from build123d import *

# Parameters (mm, degrees)
F2_T = -1
F3_R = 1


with BuildPart() as f1:
    # F0 (on Front) → F1 (revolve)
    with BuildSketch(Plane.XZ):
        Polygon((0, 9), (0, 0), (6.5, 0), (3.5, 9), align=None)
    revolve(axis=Axis((0, 0, 4.5), (0, 0, -1)))

    # F2
    f2_openings = [f1.faces().sort_by_distance(p)[0] for p in [
        (0, 0, 0),
    ]]
    offset(amount=F2_T, openings=f2_openings)

    # F3
    f3_edges = [f1.edges().sort_by_distance(p)[0] for p in [
        (-3.5, 0, 9),
    ]]
    fillet(f3_edges, radius=F3_R)


solid = f1.part
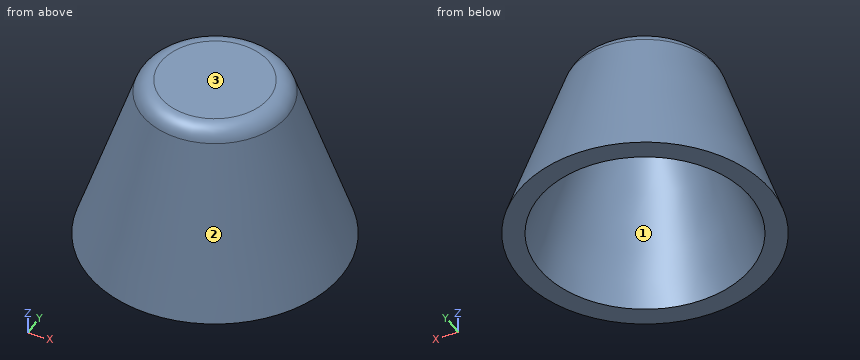
Could you check a few things on this model? Use its own coordinates, in mm. Face numbers are marked on the shaded views. Round coordinates to 2 decimals unless told otherwise and drop trailing zeros. Write each loop counter-clockwise with the first axis right and the second up, starting at its lowest first coordinate (ties: lowest second). Pieces come first, ordered by that corner, then holes. Notation, with made-up numbers: (39, -34.5) - (52, -34.5) arc R16 cw to (52, -8.5) - close; hole circle Ø7 at (-25.75, -1.5). An arc over 180 degrees is marked (long way). Use a Markdown table: item, result.
Q1. I want a section at A-A (x = 0). List the corners of the cut face in (y, z) for me.
Output values:
| item | result |
|---|---|
| outline | (-6.5, 0) - (-5.45, 0) - (-2.78, 8) - (2.78, 8) - (5.45, 0) - (6.5, 0) - (3.73, 8.32) arc R1 ccw to (2.78, 9) - (-2.78, 9) arc R1 ccw to (-3.73, 8.32) - close |
Q2. For pin 1 (1.5 mm diameter, centred on y = 1, z = 3.5, fed in from +X); pin 2 (1 mm diameter, centred on x = 5, z = 3, fed in from +Y); pin 3 (6 mm diameter, centred on x = -3.5, y = -2.5, fed in from +Z); pin 4 (1.7 mm diameter, centred on x = 1, y = 1.5, fed in from -Z), each with a flat end and sliding along its axis, tell me the tip position at first contact or that it passes through.
Output values:
| item | result |
|---|---|
| pin 1 | x = 5.52 |
| pin 2 | y = 3.22 |
| pin 3 | z = 9 |
| pin 4 | z = 8 |
Q3. Thinking about a two-plate mould opening in Y: for the marked faces 1, 2 and 3, which applies, released by +Y, released by -Y, zero draft, split by the parting line, or undercut?
Output values:
| item | result |
|---|---|
| face 1 | undercut |
| face 2 | split by the parting line |
| face 3 | zero draft |
Q4. I want a section at C-C (z = 1.25). List the corners of the cut face in (x, y) for me, plus the area to 3 significant figures.
Output values:
| item | result |
|---|---|
| outline | circle Ø12.17 at (0, 0); hole circle Ø10.06 at (0, 0) |
| area | 36.8 mm2 |
Q5. I want a section at D-D (z = 5). List the corners of the cut face in (x, y) for me.
Output values:
| item | result |
|---|---|
| outline | circle Ø9.67 at (0, 0); hole circle Ø7.56 at (0, 0) |
Q6. Please list where these lines run through material, in increasing order: L1, parallel to Y at x = -1.5, z = 7.25; L2, parallel to Y at x = -2, z = 0.75; L3, parallel to X at y = 2, z = 4.5.
Output values:
| item | result |
|---|---|
| L1 | -3.8 to -2.63, 2.63 to 3.8 |
| L2 | -5.92 to -4.8, 4.8 to 5.92 |
| L3 | -4.58 to -3.4, 3.4 to 4.58 |
